from build123d import *

# Parameters (mm, degrees)
F2_DEPTH = 76.2
F3_W     = 12.7
F3_H     = 50.8
F4_DEPTH = 3.175
F6_DEPTH = 12.7


with BuildPart() as f2:
    # F1 (on Top) → F2 (new body)
    with BuildSketch(Plane.XY):
        Polygon((-44.45, 3.175), (-44.45, 0), (44.45, 0), (44.45, 3.175), (41.275, 3.175), align=None)
        Polygon((41.275, 3.175), (44.45, 3.175), (44.45, 88.9), (41.275, 85.659533), align=None)
        Polygon((-19.318937, 23.816169), (41.275, 85.659533), (41.275, 88.9), (-19.341729, 28.283271), (-21.586793, 26.038207), align=None)
        Polygon((-21.586793, 26.038207), (-19.341729, 28.283271), (-26.525934, 35.467476), (-19.790742, 42.202668), (-22.035806, 44.447732), (-31.016062, 35.467476), align=None)
        Polygon((41.275, 85.659533), (44.45, 88.9), (41.275, 88.9), align=None)
    extrude(amount=F2_DEPTH)

    # F3 (on face) → F4 (cut)
    with BuildSketch(Plane(origin=(-33.241769, 33.241769, 0), x_dir=(-0.707107, -0.707107, 0), z_dir=(-0.707107, 0.707107, 0))):
        with Locations((-9.497625, 38.1)):
            Rectangle(F3_W, F3_H)
    extrude(amount=-F4_DEPTH, mode=Mode.SUBTRACT)

    # F5 (on face) → F6 (cut)
    with BuildSketch(Plane.YZ.offset(44.45)):
        with BuildLine():
            ThreePointArc((44.45, 15.875), (60.165448, 22.384552), (66.675, 38.1))
            ThreePointArc((66.675, 38.1), (60.165448, 53.815448), (44.45, 60.325))
            Line((44.45, 60.325), (44.45, 15.875))
        make_face()
        with BuildLine():
            Line((44.45, 15.875), (44.45, 60.325))
            ThreePointArc((44.45, 60.325), (22.225, 38.1), (44.45, 15.875))
        make_face()
    extrude(amount=-F6_DEPTH, mode=Mode.SUBTRACT)


solid = f2.part
CAD build for the part. Positions are in the model's coordinates, mm. A direction names the side the tool comes from. Round coordinates to 2 decimals unless told otherwise and drop trailing zeros. Order: outer loops, then holes, each group sorted by start corner. A loop starts at its lowest first (then second) coordinate and runs counter-clockwise, first axis right, second up. Notation, with made-up numbers: (-19, 61.5) -> (27, 61.5) arc R38 ccw to (27, 99.5) -> close; hole circle Ø2 at (60.25, 31.25). An arc over 180 degrees is marked (long way). Write item = value, one per line. Start each with the question number.
(1) Which spindle directions (+Z, -Z, +X, -X, +Y, -Y) get a long thin tool onto all of the face, cutting with end or side? Do faces 4 (the flat face through (-20.9, 43.31, 6.26)), 5 (the flat face through (-1, 0, 38)), 6 (the flat face through (-25, 39, 63.5)), 7 (the flat face through (-22.884, 31.825, 37.567)), 8 (the flat face through (-25.32, 29.77, 37.57)). Say none if no direction does.
(2) Pull direction Z, two halves, no side cores. Call faces 1 (the flat face through (0, 45, 0)), 2 (the flat face through (-1, 3.175, 38)), 3 (the flat face through (-27.633, 34.361, 38.456)): released by +Z, released by -Z, zero draft, split by the parting line, or undercut.
(3) Cut at A-A, the plane y = 56. List the corners of the cut face in (x, z) (3 decimals), then the cut area to 3 significant figures.
(4) Cut at C-C, the plane y = 39. List the corners of the cut face in (x, z) (3 decimals), then the cut area to 3 significant figures.
(5) Cut at D-D, the plane z = 34. List the corners of the cut face in (x, y) (3 decimals).
(6) Pin check, flat tips, straight feed: P1, Ø5, axis at x = 34.5, z = 52.5, coming from the +Y side (3 decimals); P2, Ø1.5, axis at y = 39.5, z = 47, coming from the -X side (3 decimals); P3, Ø1, axis at y = 23.5, z = 66.5, coming from the -X side. Stop position of each tip, or through.
(7) Probe line 1 (X direction, y = 34, z = 3) (3 decimals); line 2 (Y direction, x = 2, z = 4) (3 decimals); line 3 (Y direction, x = -5, z = 70) (3 decimals). List the from-to ranges inside material, lowest first. Write a range as [from, to].
(8) Cut at B-B, the plane x = -15. List the corners of the cut face in (y, z) (3 decimals), then the cut area to 3 significant figures.
Model answer:
q1.face_4 = +Z, -Z, +Y
q1.face_5 = +Z, -Z, +X, -X, -Y
q1.face_6 = -X, +Y
q1.face_7 = +Z, -Z
q1.face_8 = +Z, -Z, -X
q2.face_1 = released by -Z
q2.face_2 = zero draft
q2.face_3 = undercut
q3.outline = (8.375, 0) -> (12.215, 0) -> (12.215, 76.2) -> (8.375, 76.2) -> close; (41.275, 0) -> (44.45, 0) -> (44.45, 19.112) -> (41.275, 19.112) -> close; (41.275, 57.088) -> (44.45, 57.088) -> (44.45, 76.2) -> (41.275, 76.2) -> close
q3.area = 414 mm2
q4.outline = (-27.484, 0) -> (-22.993, 0) -> (-22.993, 12.7) -> (-27.484, 12.7) -> close; (-27.484, 63.5) -> (-22.993, 63.5) -> (-22.993, 76.2) -> (-27.484, 76.2) -> close; (-8.625, 0) -> (-4.442, 0) -> (-4.442, 76.2) -> (-8.625, 76.2) -> close; (41.275, 0) -> (44.45, 0) -> (44.45, 16.554) -> (41.275, 16.554) -> close; (41.275, 59.646) -> (44.45, 59.646) -> (44.45, 76.2) -> (41.275, 76.2) -> close
q4.area = 538 mm2
q5.outline = (-44.45, 0) -> (44.45, 0) -> (44.45, 22.606) -> (41.275, 22.606) -> (41.275, 3.175) -> (-44.45, 3.175) -> close; (-28.771, 33.222) -> (-21.587, 26.038) -> (-19.319, 23.816) -> (41.275, 85.66) -> (41.275, 66.294) -> (44.45, 66.294) -> (44.45, 88.9) -> (41.275, 88.9) -> (-19.342, 28.283) -> (-26.526, 35.467) -> close
q6.P1 = 84.625
q6.P2 = -8.875
q6.P3 = -19.51
q7.line_1 = [-29.549, -25.058], [-13.625, -9.341], [41.275, 44.45]
q7.line_2 = [0, 3.175], [45.575, 49.625]
q7.line_3 = [0, 3.175], [38.43, 42.625]
q8.outline = (0, 0) -> (3.175, 0) -> (3.175, 76.2) -> (0, 76.2) -> close; (28.224, 0) -> (32.625, 0) -> (32.625, 76.2) -> (28.224, 76.2) -> close
q8.area = 577 mm2
